```python
from build123d import *

# Parameters (mm, degrees)
SKETCH_1_R      = 2
SKETCH_1_R_2    = 4.03
EXTRUDE_1_DEPTH = 4


with BuildPart() as part:
    # 草图1 → 凸台-拉伸1 (new body)
    with BuildSketch(Plane.XY):
        with BuildLine():
            Line((2.282857143, -22.113571429), (-1.717142857, -22.113571429))
            Line((-1.717142857, -22.113571429), (-1.717142857, -31.613571429))
            Line((-1.717142857, -31.613571429), (-5.717142857, -31.613571429))
            Line((-5.717142857, -31.613571429), (-5.717142857, -39.613571429))
            Line((-5.717142857, -39.613571429), (-1.717142857, -39.613571429))
            Line((-1.717142857, -39.613571429), (13.282857143, -39.613571429))
            Line((13.282857143, -39.613571429), (126.011390324, 69.318874641))
            ThreePointArc((126.011390324, 69.318874641), (127.911107543, 87.182824703), (110.66398275, 92.20938652))
            Line((110.66398275, 92.20938652), (13.282857143, 49.538084372))
            Line((13.282857143, 49.538084372), (-1.717142857, 49.538084372))
            Line((-1.717142857, 49.538084372), (-1.717142857, 40.886428571))
            Line((-1.717142857, 40.886428571), (2.282857143, 40.886428571))
            Line((2.282857143, 40.886428571), (2.282857143, 42.236428571))
            Line((2.282857143, 42.236428571), (4.882857143, 42.236428571))
            Line((4.882857143, 42.236428571), (4.882857143, 40.886428571))
            Line((4.882857143, 40.886428571), (6.882857143, 40.886428571))
            Line((6.882857143, 40.886428571), (6.882857143, 37.886428571))
            Line((6.882857143, 37.886428571), (4.882857143, 37.886428571))
            Line((4.882857143, 37.886428571), (4.882857143, 36.536428571))
            Line((4.882857143, 36.536428571), (2.282857143, 36.536428571))
            Line((2.282857143, 36.536428571), (2.282857143, 37.886428571))
            Line((2.282857143, 37.886428571), (-1.717142857, 37.886428571))
            Line((-1.717142857, 37.886428571), (-1.717142857, 28.386428571))
            Line((-1.717142857, 28.386428571), (-5.717142857, 28.386428571))
            Line((-5.717142857, 28.386428571), (-5.717142857, 20.386428571))
            Line((-5.717142857, 20.386428571), (-1.717142857, 20.386428571))
            Line((-1.717142857, 20.386428571), (-1.717142857, 10.886428571))
            Line((-1.717142857, 10.886428571), (2.282857143, 10.886428571))
            Line((2.282857143, 10.886428571), (2.282857143, 12.236428571))
            Line((2.282857143, 12.236428571), (4.882857143, 12.236428571))
            Line((4.882857143, 12.236428571), (4.882857143, 10.886428571))
            Line((4.882857143, 10.886428571), (6.882857143, 10.886428571))
            Line((6.882857143, 10.886428571), (6.882857143, 7.886428571))
            Line((6.882857143, 7.886428571), (4.882857143, 7.886428571))
            Line((4.882857143, 7.886428571), (4.882857143, 6.536428571))
            Line((4.882857143, 6.536428571), (2.282857143, 6.536428571))
            Line((2.282857143, 6.536428571), (2.282857143, 7.886428571))
            Line((2.282857143, 7.886428571), (-1.717142857, 7.886428571))
            Line((-1.717142857, 7.886428571), (-1.717142857, -1.613571429))
            Line((-1.717142857, -1.613571429), (-5.717142857, -1.613571429))
            Line((-5.717142857, -1.613571429), (-5.717142857, -9.613571429))
            Line((-5.717142857, -9.613571429), (-1.717142857, -9.613571429))
            Line((-1.717142857, -9.613571429), (-1.717142857, -19.113571429))
            Line((-1.717142857, -19.113571429), (2.282857143, -19.113571429))
            Line((2.282857143, -19.113571429), (2.282857143, -17.763571429))
            Line((2.282857143, -17.763571429), (4.882857143, -17.763571429))
            Line((4.882857143, -17.763571429), (4.882857143, -19.113571429))
            Line((4.882857143, -19.113571429), (6.882857143, -19.113571429))
            Line((6.882857143, -19.113571429), (6.882857143, -22.113571429))
            Line((6.882857143, -22.113571429), (4.882857143, -22.113571429))
            Line((4.882857143, -22.113571429), (4.882857143, -23.463571429))
            Line((4.882857143, -23.463571429), (2.282857143, -23.463571429))
            Line((2.282857143, -23.463571429), (2.282857143, -22.113571429))
        make_face()
        with Locations((32.050124236, 25.489798741)):
            Circle(SKETCH_1_R, mode=Mode.SUBTRACT)
        with Locations((74.16649069, 52.438113656)):
            Circle(SKETCH_1_R, mode=Mode.SUBTRACT)
        with Locations((116.282857143, 79.386428571)):
            Circle(SKETCH_1_R_2, mode=Mode.SUBTRACT)
    extrude(amount=EXTRUDE_1_DEPTH)


solid = part.part
```
For this review, take the finished solid that the model builds, in its own axes (mm). A direction names the side the tool comes from. Coordinates: 2 decimals unless noted, no trailing zeros. Write each loop counter-clockwise with the first axis right and the second up, starting at its lowest first coordinate (ties: lowest second). Pieces come first, ordered by that corner, then holes. Notation, with made-up numbers: (10, 47.25) - (51, 47.25) arc R19 ccw to (51, 66.25) - close; hole circle Ø9 at (33.5, -5.5). An arc over 180 degrees is marked (long way). Answer in a Markdown table with one row per item. Add a question column.
Q1. Draft analysis for pull direction Y (two halves, no side actions). For faces 1 (the flat face through (-1.717, 16, 2)), 2 (the flat face through (6, 49.538, 2)), 3 (the flat face through (46, 28, 4)), state which applies: +Y half, -Y half, draft (parallel to the pull), parting line (faces both ways), or undercut.
Q2. We need section C-C, the plane x = 60.5. State the section outline as (y, z) points, and give its area (3 significant figures).
Q3. We need section B-B, the plane y = -30. State the section outline as (x, z) points.
Q4. For probe 1 along Y at (x, z) = (114.5, 3.75); probe 2 along X at (y, z) = (51.5, 1.4); probe 3 along Y at (x, z) = (113.5, 1), list the stretches that pass through material, from the lowest coordinate up.
Q5. Tool access review of faces 4 (the flat face through (-4, 28.386, 2)), 5 (the flat face through (0, 37.886, 2)), 6 (the flat face through (46, 28, 0)): name each direction out of +Z, -Z, +X, -X, +Y, -Y from which nothing blocks a thin tool from reaching the whole face with its end or side.
Q6. We need section D-D, the plane z = 1.15. Count the separate pieces of the cut face and the enclosed holes in it, and give its area (3 significant figures).
Q7. For P1, Ø6, axis at x = 45.5, y = 43, coming from the -Z side; P2, Ø1.1, axis at y = -19, z = 3, coming from the -X side; P3, Ø1, axis at x = 6, z = 2, coming from the +Y side; P4, Ø1.5, axis at y = 73, z = 1, coming from the -X side, all flat-tipped, find the tip position at first contact; note any pin that passes through.
Q8. We need section A-A, the plane x = 118. State the section outline as (y, z) points.
Answer list:
| question | item | result |
|---|---|---|
| 1 | face 1 | undercut |
| 1 | face 2 | +Y half |
| 1 | face 3 | draft |
| 2 | outline | (6.01, 0) - (70.23, 0) - (70.23, 4) - (6.01, 4) - close |
| 2 | area | 257 mm2 |
| 3 | outline | (-1.72, 0) - (23.23, 0) - (23.23, 4) - (-1.72, 4) - close |
| 4 | probe 1 | y = 58.2 to 75.77, 83 to 93.27 |
| 4 | probe 2 | x = 17.76 to 72.4, 75.93 to 107.57 |
| 4 | probe 3 | y = 57.23 to 76.47, 82.3 to 93.11 |
| 5 | face 4 | +Z, -Z, -X, +Y |
| 5 | face 5 | +Z, -Z, -X |
| 5 | face 6 | -Z, +X, -X, +Y, -Y |
| 6 | separate pieces | 1 |
| 6 | enclosed holes | 3 |
| 6 | area | 7,960 mm2 |
| 7 | P1 | stops at z = 0 |
| 7 | P2 | stops at x = -1.72 |
| 7 | P3 | stops at y = 49.54 |
| 7 | P4 | stops at x = 65.11 |
| 8 | outline | (61.58, 0) - (75.74, 0) - (75.74, 4) - (61.58, 4) - close; (83.03, 0) - (93.28, 0) - (93.28, 4) - (83.03, 4) - close |
